```python
from build123d import *

# Parameters (mm, degrees)
CROQUIS1_W                = 10
CROQUIS1_H                = 10
CROQUIS1_R                = 1.625
SALIENTE_EXTRUIR1_DEPTH   = 3
SALIENTE_EXTRUIR1_2_DEPTH = 3
CROQUIS2_W                = 40
CROQUIS2_H                = 10
CROQUIS2_R                = 1
SALIENTE_EXTRUIR2_DEPTH   = 3
SALIENTE_EXTRUIR3_START   = 5
CROQUIS3_R                = 3
CROQUIS3_R_2              = 1
SALIENTE_EXTRUIR3_DEPTH   = 5
CHAFL_N1_SIZE             = 2
CHAFL_N2_SIZE             = 21


with BuildPart() as part:
    # Croquis1 → Saliente-Extruir1 (new body)
    with BuildSketch(Plane.XY):
        Rectangle(CROQUIS1_W, CROQUIS1_H)
        Circle(CROQUIS1_R, mode=Mode.SUBTRACT)
    extrude(amount=SALIENTE_EXTRUIR1_DEPTH)



with BuildPart() as body_2:
    # Croquis1 → Saliente-Extruir1 2 (new body)
    with BuildSketch(Plane.XY):
        with Locations((-50, 0)):
            Rectangle(CROQUIS1_W, CROQUIS1_H)
        with Locations((-50, 0)):
            Circle(CROQUIS1_R, mode=Mode.SUBTRACT)
    extrude(amount=SALIENTE_EXTRUIR1_2_DEPTH)


with BuildPart() as part_1:
    add(part.part)

    add(body_2.part)  # Saliente-Extruir2 merges body 2
    # Croquis2 → Saliente-Extruir2 (add)
    # profile 1 of 2: a face of its own
    with BuildSketch(Plane.XY.offset(3)):
        with Locations((-25, 0)):
            Rectangle(CROQUIS2_W, CROQUIS2_H)
        with Locations((-15, 0)):
            Circle(CROQUIS2_R, mode=Mode.SUBTRACT)
    # profile 2 of 2: a face of its own
    with BuildSketch(Plane.XY.offset(3)):
        Polygon((-61, -5), (-61, -26), (-71, -26), (-71, 26), (-61, 26), (-61, 5), (-55, 5), (-55, -5), align=None)
        with Locations((-66, 21)):
            Circle(CROQUIS2_R, mode=Mode.SUBTRACT)
        with Locations((-66, -21)):
            Circle(CROQUIS2_R, mode=Mode.SUBTRACT)
    extrude(amount=-SALIENTE_EXTRUIR2_DEPTH)

    # Croquis3 → Saliente-Extruir3 (add)
    # profile 1 of 3: a face of its own
    with BuildSketch(Plane.XY.offset(3).offset(SALIENTE_EXTRUIR3_START)):
        with Locations((-66, 21)):
            Circle(CROQUIS3_R)
        with Locations((-66, 21)):
            Circle(CROQUIS3_R_2, mode=Mode.SUBTRACT)
    # profile 2 of 3: a face of its own
    with BuildSketch(Plane.XY.offset(3).offset(SALIENTE_EXTRUIR3_START)):
        with Locations((-66, -21)):
            Circle(CROQUIS3_R)
        with Locations((-66, -21)):
            Circle(CROQUIS3_R_2, mode=Mode.SUBTRACT)
    # profile 3 of 3: a face of its own
    with BuildSketch(Plane.XY.offset(3).offset(SALIENTE_EXTRUIR3_START)):
        with Locations((-15, 0)):
            Circle(CROQUIS3_R)
        with Locations((-15, 0)):
            Circle(CROQUIS3_R_2, mode=Mode.SUBTRACT)
    extrude(amount=-SALIENTE_EXTRUIR3_DEPTH)

    # Chaflán1
    chafl_n1_edges = [part_1.edges().sort_by_distance(p)[0] for p in [
        (-69, 21, 3),
        (-69, -21, 3),
        (-18, 0, 3),
    ]]
    chamfer(chafl_n1_edges, length=CHAFL_N1_SIZE - 0.0001)  # a hair under: the kernel refuses the full size

    # Chaflán2
    chafl_n2_edges = [part_1.edges().sort_by_distance(p)[0] for p in [
        (-61, 5, 1.5),
        (-61, -5, 1.5),
    ]]
    chamfer(chafl_n2_edges, length=CHAFL_N2_SIZE - 0.0001)  # a hair under: the kernel refuses the full size


solid = part_1.part
```
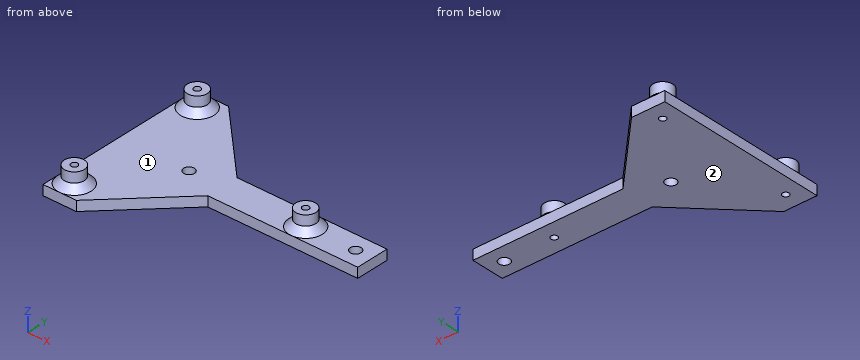
CAD build for the part. Positions are in the model's coordinates, mm. Face numbers are marked on the shaded views. Round coordinates to 2 decimals unless told otherwise and drop trailing zeros. Write each loop counter-clockwise with the first axis right and the second up, starting at its lowest first coordinate (ties: lowest second). Pieces come first, ordered by that corner, then holes. Notation, with made-up numbers: (82.5, 22.25) -> (95.5, 22.25) arc R23 ccw to (95.5, 33.25) -> close; hole circle Ø6 at (20, -17). An arc over 180 degrees is marked (long way). Answer in a Markdown table with one row per item. Add a question column.
Item 1: Mould opens along Y. For the marked faces 1 and 2 say: pulls with the +Y half, pulls with the -Y half, needs draft (parallel to the pull), parting line crosses it, or undercut.
Item 2: Saw through at A-A, the plane x = -66. Count the separate pieces of the cut face and the enclosed holes in it, then the cut area to 3 significant figures.
Item 3: Drop flat-ended pins along their axis: pin 1 Ø2.5 at (x, y) = (0, 0) entering from -Z; pin 2 Ø0.9 at (x, z) = (-24, 1.5) entering from -Y; pin 3 Ø3.5 at (x, z) = (-15, 2) entering from +Y. Give the stop position or say it passes through.
Item 4: Drill centre lines: line 1 (Y direction, x = -15, z = 5.25); line 2 (Y direction, x = 0, z = 2) (3 decimals); line 3 (Z direction, x = -8.5, y = -2.5). Where is each one in solid material? Low to high. Write a range as from..to.
Item 5: Saw through at B-B, the plane z = 6.5. Write the cut outline in (x, y).
Findings below:
| question | item | result |
|---|---|---|
| 1 | face 1 | undercut |
| 1 | face 2 | needs draft |
| 2 | separate pieces | 3 |
| 2 | enclosed holes | 0 |
| 2 | area | 192 mm^2 |
| 3 | pin 1 | passes through |
| 3 | pin 2 | stops at y = -5 |
| 3 | pin 3 | stops at y = 5 |
| 4 | line 1 | y = -3..-1, 1..3 |
| 4 | line 2 | y = -5..-1.625, 1.625..5 |
| 4 | line 3 | z = 0..3 |
| 5 | outline | circle Ø6 at (-66, -21); circle Ø6 at (-66, 21); circle Ø6 at (-15, 0); hole circle Ø2 at (-66, -21); hole circle Ø2 at (-66, 21); hole circle Ø2 at (-15, 0) |
